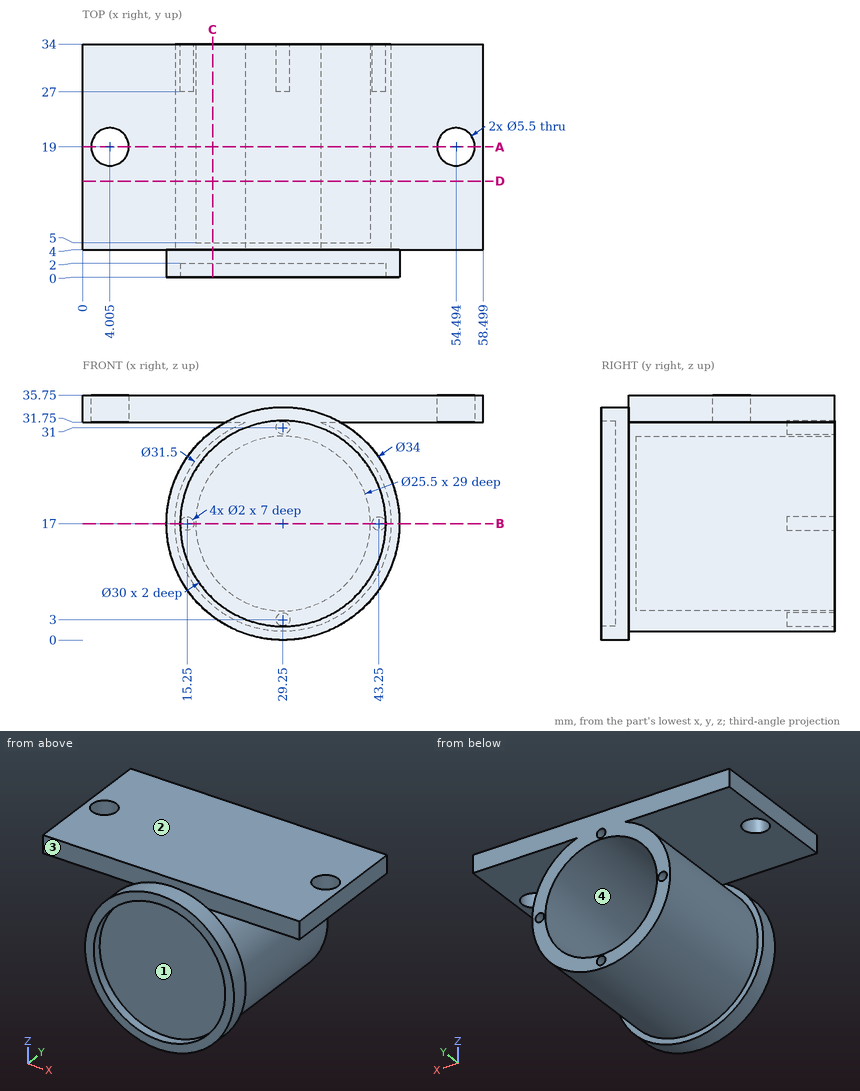
Design review of the part shown in the three views and the two pictorial views. Dimensions are in mm from the part's minimum x, y and z. A direction names the side the tool comes from. Give positions to 0.01 mm unless a question says otherwise; leave off trailing zeros. Order: outer loops, then holes, each group sorted by start corner. A loop starts at its lowest first (then second) coordinate and runs counter-clockwise, first axis right, second up. Notation, with made-up numbers: (23, 11.5) -> (48, 11.5) arc R16 ccw to (48, 28.5) -> close; hole circle Ø10 at (5.5, 35). An arc over 180 degrees is marked (long way). Write each question's results on one line, items separated by ' | '. Start each with the question number.
Q1. Add section C-C on x = 19. Give the boundary of the cut face in (y, z).
Q2. Add section B-B on z = 17. Give the boundary of the cut face in (x, y).
Q3. Add section A-A on y = 19. State how many separate pieces and enclosed holes the cut face has, and give its area (3 significant figures).
Q4. Wall thickness on L1, parallel to X at y = 30.25, z = 17; L2, parallel to X at y = 11.25, z = 17; L3, parallel to Z at x = 36.5, y = 9.5: over which ranges is each line inside the solid? List them lowest first. Write a range as from..to.
Q5. Machinability: for the marked faces 1, 2, 3 and 4, which of the approach directions +Z, -Z, +X, -X, +Y, -Y give a long, thin tool a straight path to every point of the face, cutting with its end or side? Answer none if there is none.
Q6. Add section D-D on y = 14. Give the boundary of the cut face in (x, z).
Q7. For pin 1 (4.5 mm diameter, centred on x = 4, y = 19, fed in from +Z); pin 2 (4 mm diameter, centred on y = 4, z = 12, fed in from +X); pin 3 (1.6 mm diameter, centred on x = 29.25, z = 31, fed in from -Y); pin 4 (1 mm diameter, centred on x = 18.5, y = 9, fed in from -Z), all flat-tipped, find the tip position at first contact; note any pin that passes through.
Found:
1) outline: (0, 3.44) -> (4, 3.44) -> (4, 5.04) -> (34, 5.04) -> (34, 9.42) -> (5, 9.42) -> (5, 24.58) -> (34, 24.58) -> (34, 28.96) -> (4, 28.96) -> (4, 30.56) -> (0, 30.56) -> (0, 27.95) -> (2, 27.95) -> (2, 6.05) -> (0, 6.05) -> close; (4, 31.75) -> (34, 31.75) -> (34, 35.75) -> (4, 35.75) -> close
2) outline: (12.25, 0) -> (14.25, 0) -> (14.25, 2) -> (44.25, 2) -> (44.25, 0) -> (46.25, 0) -> (46.25, 4) -> (45, 4) -> (45, 34) -> (44.25, 34) -> (44.25, 27) -> (42.25, 27) -> (42.25, 34) -> (42, 34) -> (42, 5) -> (16.5, 5) -> (16.5, 34) -> (16.25, 34) -> (16.25, 27) -> (14.25, 27) -> (14.25, 34) -> (13.5, 34) -> (13.5, 4) -> (12.25, 4) -> close
3) separate pieces: 3 | enclosed holes: 1 | area: 451 mm2
4) L1: x = 13.5..14.25, 16.25..16.5, 42..42.25, 44.25..45 | L2: x = 13.5..16.5, 42..45 | L3: z = 3.02..6.51, 27.49..30.98, 31.75..35.75
5) face 1: -Y | face 2: +Z, +X, -X, +Y, -Y | face 3: +Z, -Y | face 4: +Y
6) outline: (0, 31.75) -> (23.73, 31.75) arc R15.75 ccw (long way) to (34.77, 31.75) -> (58.5, 31.75) -> (58.5, 35.75) -> (0, 35.75) -> close; hole circle Ø25.5 at (29.25, 17)
7) pin 1: passes through | pin 2: stops at x = 45.98 | pin 3: stops at y = 2 | pin 4: stops at z = 5.04
